Could you check a few things on this model? Use its own coordinates, in mm. A direction names the side the tool comes from. Coordinates: 2 decimals unless noted, no trailing zeros. Write each loop counter-clockwise with the first axis right and the second up, starting at its lowest first coordinate (ties: lowest second). Pieces come first, ordered by that corner, then holes. Notation, with made-up numbers: M -0.5,32 L 50.5,32 A18 ccw 50.5,45 Z; hole C -15.5,0 d1. An arc over 180 degrees is marked long. Write item = value, one per line.
Solid Edge part; units mm, degrees
sketch "Sketch1" plane through (0, 0, 0) normal (0, 0, 1) x (1, 0, 0)
  circle A0 centre (0, 0) radius 3.5
extrude "Protrusion1" add sketch "Sketch1" along normal blind 4
sketch "Sketch2" plane through (0, 0, 0) normal (0, 0, -1) x (1, 0, 0)
  circle A0 centre (0, 0) radius 2
extrude "Protrusion2" add sketch "Sketch2" along normal blind 6
sketch "Sketch3" plane through (0, 0, -6) normal (0, 0, -1) x (1, 0, 0)
  circle A0 centre (0, 0) radius 1.9997
extrude "Cutout1" cut sketch "Sketch3" against normal blind 5.994 flip side to cut
chamfer "Chamfer_1" distance 0.3 angle 45 1 edges at (-1.9997, 0, -6)
sketch "Sketch4" plane through (0, 0, 4) normal (0, 0, 1) x (1, 0, 0)
  line L0 (-0.866, 1.5) -> (0.866, 1.5)
  line L1 (1.7321, 0) -> (0.866, 1.5)
  line L2 (0.866, -1.5) -> (1.7321, 0)
  line L3 (-0.866, -1.5) -> (0.866, -1.5)
  line L4 (-1.7321, 0) -> (-0.866, -1.5)
  line L5 (-0.866, 1.5) -> (-1.7321, 0)
extrude "Cutout2" cut sketch "Sketch4" against normal blind 2
properties part number "185699" material "Stainless Steel, 304"
Item 1: If we mould it in two halves opening along Y, with no side actions, what happens to faces 4 (the face through (3.233, 1.341, 1.972)), 5 (the face through (0, -2, 4)), 6 (the face through (-1.305, -0.74, 3.014))? For each: pulls with the +Y half, pulls with the -Y half, needs draft (parallel to the pull), parting line crosses it, or undercut.
Numbers:
face_4 = parting line crosses it
face_5 = needs draft
face_6 = undercut
Item 2: Imagine slicing it at A-A (z = 3). Write out the boundary of the cut face in (x, y), and give its area (3 significant figures).
Numbers:
outline = C 0,0 d7; hole M -1.73,0 L -0.87,-1.5 L 0.87,-1.5 L 1.73,0 L 0.87,1.5 L -0.87,1.5 Z
area = 30.7 mm²
Item 3: If I drill on line 1 along Y through (x, z) = (-1, -0.25); line 2 along X through (y, z) = (0, -4.5); line 3 along Z through (x, y) = (-1.5, 2.5), over which ranges is the centre line in solid material (lowest first)?
Numbers:
line_1 = -1.73 to 1.73
line_2 = -2 to 2
line_3 = 0 to 4
Item 4: I'm going to push flat-ended pins straight in: P1, Ø2, axis at y = -1.5, z = 2, coming from the -X side; P2, Ø4, axis at y = -0.5, z = -4.5, coming from the -X side; P3, Ø1.5, axis at x = -2.5, z = -1, coming from the -Y side. Where does each tip first touch, or does it pass through?
Numbers:
P1 = -3.46
P2 = -2
P3 = -0.97
Item 5: Imagine slicing it at C-C (z = 0.75). Write out the boundary of the cut face in (x, y), and give its area (3 significant figures).
Numbers:
outline = C 0,0 d7
area = 38.5 mm²
Item 6: Imagine slicing it at D-D (y = 2.25). Write out the boundary of the cut face in (x, z).
Numbers:
outline = M -2.68,0 L 2.68,0 L 2.68,4 L -2.68,4 Z
Item 7: For faces 1 (the face through (0, 1.5, 3)), 2 (the face through (0, 0, -6)), 3 (the face through (2, -2, 0)), which set-ups out of +Z, -Z, +X, -X, +Y, -Y let a thin tool reach every point of the face, with its end or its side?
Numbers:
face_1 = +Z
face_2 = -Z, +X, -X, +Y, -Y
face_3 = -Z
